Input: part model. Units: mm. Frame: model coordinates. A direction names the side the tool comes from. Give positions to 0.01 mm unless a question says otherwise; leave off trailing zeros. Loops run counter-clockwise (first coordinate to the right, second up) from the corner with the lowest first, then second, coordinate; pieces in that order, holes last. Notation, with made-up numbers: (82, -28.5) - (93, -28.5) arc R13 ccw to (93, -12.5) - close; hole circle Ø7 at (-37, 70). An arc over 180 degrees is marked (long way). One line per item, written item: value.
from build123d import *

# Parameters (mm, degrees)
EXTRUDE_1_DEPTH     = 6
SKETCH_2_R          = 1.65
CUT_EXTRUDE_1_DEPTH = 171.71260254


with BuildPart() as part:
    # Эскиз1 → Бобышка-Вытянуть1 (new body)
    with BuildSketch(Plane.XY):
        Polygon((-164.468308742, 1.015256317), (-164.468308742, -37.946418867), (-59.578582118, -37.946418867), (-21.632163251, 0), (84.510530021, 0), (84.510530021, 15.353810043), (90.710530021, 15.353810043), (90.710530021, 25.353810043), (84.510530021, 25.353810043), (84.510530021, 35.353810043), (90.710530021, 35.353810043), (90.710530021, 45.353810043), (45.113947205, 45.353810043), (45.113947205, 39.153810043), (20.113947205, 39.153810043), (20.113947205, 45.353810043), (-4.886052795, 45.353810043), (-4.886052795, 39.153810043), (-29.886052795, 39.153810043), (-29.886052795, 45.353810043), (-54.886052795, 45.353810043), (-54.886052795, 23.298924803), (-77.169721281, 1.015256317), align=None)
    extrude(amount=EXTRUDE_1_DEPTH)

    # Эскиз2 → Вырез-Вытянуть1 (cut, through all)
    with BuildSketch(Plane.XY.offset(6)):
        with Locations((-127.888308742, -3.984743683)):
            Circle(SKETCH_2_R)
        with Locations((-127.888308742, -33.984743683)):
            Circle(SKETCH_2_R)
        with BuildLine():
            Line((-157.968308742, -10.634743683), (-157.968308742, -11.984743683))
            Line((-157.968308742, -11.984743683), (-160.968308742, -11.984743683))
            Line((-160.968308742, -11.984743683), (-160.968308742, -10.634743683))
            Line((-160.968308742, -10.634743683), (-164.468308742, -10.634743683))
            Line((-164.468308742, -10.634743683), (-164.468308742, -7.334743683))
            Line((-164.468308742, -7.334743683), (-160.968308742, -7.334743683))
            Line((-160.968308742, -7.334743683), (-160.968308742, -5.984743683))
            Line((-160.968308742, -5.984743683), (-157.968308742, -5.984743683))
            Line((-157.968308742, -5.984743683), (-157.968308742, -7.334743683))
            Line((-157.968308742, -7.334743683), (-155.968308742, -7.334743683))
            ThreePointArc((-155.968308742, -7.334743683), (-154.90764857, -7.774083512), (-154.468308742, -8.834743683))
            Line((-154.468308742, -8.834743683), (-154.468308742, -9.134743683))
            ThreePointArc((-154.468308742, -9.134743683), (-154.90764857, -10.195403855), (-155.968308742, -10.634743683))
            Line((-155.968308742, -10.634743683), (-157.968308742, -10.634743683))
        make_face()
        with BuildLine():
            Line((-160.968308742, -25.984743683), (-157.968308742, -25.984743683))
            Line((-157.968308742, -25.984743683), (-157.968308742, -27.334743683))
            Line((-157.968308742, -27.334743683), (-155.968308742, -27.334743683))
            ThreePointArc((-155.968308742, -27.334743683), (-154.90764857, -27.774083512), (-154.468308742, -28.834743683))
            Line((-154.468308742, -28.834743683), (-154.468308742, -29.134743683))
            ThreePointArc((-154.468308742, -29.134743683), (-154.90764857, -30.195403855), (-155.968308742, -30.634743683))
            Line((-155.968308742, -30.634743683), (-157.968308742, -30.634743683))
            Line((-157.968308742, -30.634743683), (-157.968308742, -31.984743683))
            Line((-157.968308742, -31.984743683), (-160.968308742, -31.984743683))
            Line((-160.968308742, -31.984743683), (-160.968308742, -30.634743683))
            Line((-160.968308742, -30.634743683), (-164.468308742, -30.634743683))
            Line((-164.468308742, -30.634743683), (-164.468308742, -27.334743683))
            Line((-164.468308742, -27.334743683), (-160.968308742, -27.334743683))
            Line((-160.968308742, -27.334743683), (-160.968308742, -25.984743683))
        make_face()
    extrude(amount=-CUT_EXTRUDE_1_DEPTH, mode=Mode.SUBTRACT)


solid = part.part
Item 1: Draft query along X for faces 1 (the face through (84.511, 30, 3)), 2 (the face through (88, 25.354, 3)), 3 (the face through (33, 39.154, 3)). Return one class per face: pulls with the +X half, pulls with the -X half, needs draft (parallel to the pull), parting line crosses it, or undercut.
Verdict:
face 1: pulls with the +X half
face 2: needs draft
face 3: undercut
Item 2: Access query for faces 4 (the face through (88, 15.354, 3)), 5 (the face through (-54.886, 34, 3)), 6 (the face through (88, 35.354, 3)), 7 (the face through (-29.886, 42, 3)). Directions: +Z, -Z, +X, -X, +Y, -Y. A direction counts if a zero-diameter tool reaches every point of the face in a straight line with its end or side. Return the directions, or none.
Verdict:
face 4: +Z, -Z, +X, -Y
face 5: +Z, -Z, -X, +Y
face 6: +Z, -Z, +X
face 7: +Z, -Z, +Y
Item 3: Pin query (flat end, axial travel): P1, Ø1.8, axis at y = 29.5, z = 3, coming from the +X side; P2, Ø1, axis at x = -71, z = 2.5, coming from the +Y side (3 decimals); P3, Ø1, axis at x = -156.5, z = 3.5, coming from the +Y side. Return the tip coordinate at first contact, or that it passes through.
Verdict:
P1: stops at x = 84.51
P2: stops at y = 7.685
P3: stops at y = 1.02
Item 4: Section A-A, the plane x = -83. Output: boundary loops of the cut face in (y, z).
Verdict:
outline: (-37.95, 0) - (1.02, 0) - (1.02, 6) - (-37.95, 6) - close
Item 5: Material intervals for L1, parallel to Y at x = -0.5, z = 2.65; L2, parallel to Y at x = -81.5, z = 1.6; L3, parallel to X at y = 38, z = 3.15, sorted ascending.
Verdict:
L1: y = 0 to 45.35
L2: y = -37.95 to 1.02
L3: x = -54.89 to 90.71
Item 6: Section C-C, the plane z = 4.75. Count the separate pieces of the cut face and the enclosed holes in it, and give its area (3 significant figures).
Verdict:
separate pieces: 1
enclosed holes: 2
area: 11,100 mm^2
Item 7: Section B-B, the plane y = 6. Output: boundary loops of the cut face in (x, z), and give its area (3 significant figures).
Verdict:
outline: (-72.18, 0) - (84.51, 0) - (84.51, 6) - (-72.18, 6) - close
area: 940 mm^2
